```python
from build123d import *

# Parameters (mm, degrees)
F0_W      = 42
F0_H      = 36
F1_DEPTH  = 2
F2_R      = 2
F3_R      = 1.5
F4_DEPTH  = 2
F5_W      = 2
F5_H      = 30
F6_DEPTH  = 14
F7_W      = 2
F7_H      = 30
F8_DEPTH  = 11
F9_W      = 22
F9_H      = 36
F10_DEPTH = 2
F11_W     = 8
F11_H     = 4.9999979734
F11_H_2   = 1.0000020266
F12_DEPTH = 3
F13_R     = 1
F7_W_2    = 8
F7_H_2    = 6
F14_DEPTH = 6


# Not quite as in the source:
# - a feature names something its author has since deleted; it is built from what else it names


with BuildPart() as f1:
    # F0 (on Top) → F1 (new body)
    with BuildSketch(Plane.XY):
        with Locations((6.745641768, -5.4418604523)):
            Rectangle(F0_W, F0_H)
    extrude(amount=F1_DEPTH)

    # F2
    f2_edges = [f1.edges().sort_by_distance(p)[0] for p in [
        (27.745642, -23.44186, 1),
        (27.745642, 12.55814, 1),
        (-14.254358, -23.44186, 1),
        (-14.254358, 12.55814, 1),
    ]]
    fillet(f2_edges, radius=F2_R)

    # F3 (on face) → F4 (cut)
    with BuildSketch(Plane.XY.offset(2)):
        with Locations((-12.254358232, 10.5581395477)):
            Circle(F3_R)
        with Locations((-12.254358232, -21.4418604523)):
            Circle(F3_R)
        with Locations((25.745641768, -21.4418604523)):
            Circle(F3_R)
        with Locations((25.745641768, 10.5581395477)):
            Circle(F3_R)
    extrude(amount=-F4_DEPTH, mode=Mode.SUBTRACT)

    # F5 (on face) → F6 (join)
    with BuildSketch(Plane(origin=(0, 0, 0), x_dir=(1, 0, 0), z_dir=(0, 0, -1))):
        with Locations((16.7456435263, 5.4418606311)):
            Rectangle(F5_W, F5_H)
        with Locations((-3.2543599904, 5.4418606311)):
            Rectangle(F5_W, F5_H)
    extrude(amount=F6_DEPTH)

    # F7 (on face) → F8 (join)
    with BuildSketch(Plane.XY.offset(2)):
        with Locations((16.7456435263, -5.4418606311)):
            Rectangle(F7_W, F7_H)
        with Locations((-3.2543599904, -5.4418606311)):
            Rectangle(F7_W, F7_H)
    extrude(amount=F8_DEPTH)

    # F9 (on face) → F10 (join)
    with BuildSketch(Plane.XY.offset(13)):
        with Locations((6.7456400096, -5.4360154718)):
            Rectangle(F9_W, F9_H)
    extrude(amount=F10_DEPTH)

    # F11 (on face) → F12 (join)
    with BuildSketch(Plane.XY.offset(15)):
        with Locations((6.7456399985, -20.9360164851)):
            Rectangle(F11_W, F11_H)
        with Locations((6.7456399985, -23.9360164851)):
            Rectangle(F11_W, F11_H_2)
    extrude(amount=F12_DEPTH)

    # F13
    f13_edges = [f1.edges().sort_by_distance(p)[0] for p in [
        (10.74564, -21.436017, 18),
        (2.74564, -21.436017, 18),
    ]]
    fillet(f13_edges, radius=F13_R)

    # F7 (on face) → F14 (join)
    with BuildSketch(Plane.XY.offset(2)):
        with Locations((6.829907462, -17.511118643)):
            Rectangle(F7_W_2, F7_H_2)
    extrude(amount=F14_DEPTH)


with BuildPart() as f15_1:
    # F15: copy of F1
    add(f1.part)


solid = f1.part
```
Check sheet for the modelled part. Datum: model origin and axes. Units: mm. A direction names the side the tool comes from. Round coordinates to 2 decimals unless told otherwise and drop trailing zeros. Loops run counter-clockwise (first coordinate to the right, second up) from the corner with the lowest first, then second, coordinate; pieces in that order, holes last. Notation, with made-up numbers: (25.25, -38.75) - (36.25, -38.75) arc R36 cw to (36.25, -2.75) - close; hole circle Ø10 at (74, 50.5). An arc over 180 degrees is marked (long way). Answer as a JSON object with one key per item and string values. Group by question number.
Q1. Set-up check for faces 4 (the face through (7, -14.511, 5)), 5 (the face through (17, -20.442, 7)), 6 (the face through (15.746, -5, -7)): record each of +Z, -Z, +X, -X, +Y, -Y from which the full face is reachable in a straight line by a thin tool's end or side.
Q2. Sectioned sample at B-B, the plane x = 9. Enter the section's corners in (y, z).
Q3. Sectioned sample at D-D, the plane z = -2. Enter the section's corners in (x, y), plus the area to 3 significant figures.
Q4. Mould release check, pull along X, two halves, no side actions. Record for faces 1 (the face through (-4.254, -5, -7)), 2 (the face through (10.83, -18, 5)), 3 (the face through (7, -24, 15)): released by +X, released by -X, zero draft, split by the parting line, or undercut.
Q5. Scan lines: line 1 along Z through (x, y) = (13.5, 4); line 2 along X through (y, z) = (-9, 9.5); line 3 along Z through (x, y) = (5.5, -18). Record each from-to range of solid material in increasing order. Write a range as [from, to].
Q6. Gauge pin test, flat ends, axial feed: P1, Ø1.5, axis at y = -11, z = 4, coming from the +X side; P2, Ø3, axis at y = -1.5, z = -6, coming from the -X side; P3, Ø1, axis at x = -1.5, z = 0.5, coming from the +Y side. Record the tip position at first contact, or that the pin passes through.
Q7. Sectioned sample at A-A, the plane z = 3.5. Enter the section's corners in (x, y), plus the area to 3 significant figures.
Solution:
{
 "1": {"face 4": "+Y", "face 5": "+X, -Y", "face 6": "-Z, +Y, -Y"},
 "2": {"outline": "(-24.44, 15) - (-23.44, 15) - (-23.44, 13) - (12.56, 13) - (12.56, 15) - (-18.44, 15) - (-18.44, 18) - (-24.44, 18) - close; (-23.44, 0) - (12.56, 0) - (12.56, 2) - (-14.51, 2) - (-14.51, 8) - (-20.51, 8) - (-20.51, 2) - (-23.44, 2) - close"},
 "3": {"outline": "(-4.25, -20.44) - (-2.25, -20.44) - (-2.25, 9.56) - (-4.25, 9.56) - close; (15.75, -20.44) - (17.75, -20.44) - (17.75, 9.56) - (15.75, 9.56) - close", "area": "120 mm²"},
 "4": {"face 1": "released by -X", "face 2": "undercut", "face 3": "zero draft"},
 "5": {"line 1": "z = [0, 2], [13, 15]", "line 2": "x = [-4.25, -2.25], [15.75, 17.75]", "line 3": "z = [0, 8], [13, 15]"},
 "6": {"P1": "stops at x = 17.75", "P2": "stops at x = -4.25", "P3": "stops at y = 12.56"},
 "7": {"outline": "(-4.25, -20.44) - (-2.25, -20.44) - (-2.25, 9.56) - (-4.25, 9.56) - close; (2.83, -20.51) - (10.83, -20.51) - (10.83, -14.51) - (2.83, -14.51) - close; (15.75, -20.44) - (17.75, -20.44) - (17.75, 9.56) - (15.75, 9.56) - close", "area": "168 mm²"}
}
